For this review, take the finished solid that the model builds, in its own axes (mm). Face numbers are marked on the shaded views. A direction names the side the tool comes from. Round coordinates to 2 decimals unless told otherwise and drop trailing zeros. Loops run counter-clockwise (first coordinate to the right, second up) from the corner with the lowest first, then second, coordinate; pieces in that order, holes last.
1) Insertion check: pin 1 (1 mm diameter, centred on x = 202, y = 166.5, fed in from -Z). The pin has a flat end and moves straight along its axis. Give the tip position at first contact, or say it passes through.
2) Take a section at D-D (y = 178.25). State the section outline as (x, z) points.
3) Take a section at C-C (x = 196). State the section outline as (y, z) points.
4) Wall thickness on L1, parallel to Y at x = 202.5, z = 2.4; L2, parallel to Y at x = 195.5, z = 2.75; L3, parallel to X at y = 174.25, z = 1.45: over which ranges is each line inside the solid? List them lowest first.
5) Take a section at A-A (x = 203.5). State the section outline as (y, z) points.
6) Mouldability with a two-part tool opening along Y and no side actions: class the marked faces 3, 4, 5 and 6 as pulls with the +Y half, pulls with the -Y half, needs draft (parallel to the pull), parting line crosses it, or undercut.
7) Take a section at B-B (z = 1.1). State the section outline as (x, y) points.
8) Tool access review of the marked faces 1 and 2: name each direction out of +Z, -Z, +X, -X, +Y, -Y from which nothing blocks a thin tool from reaching the whole face with its end or side.
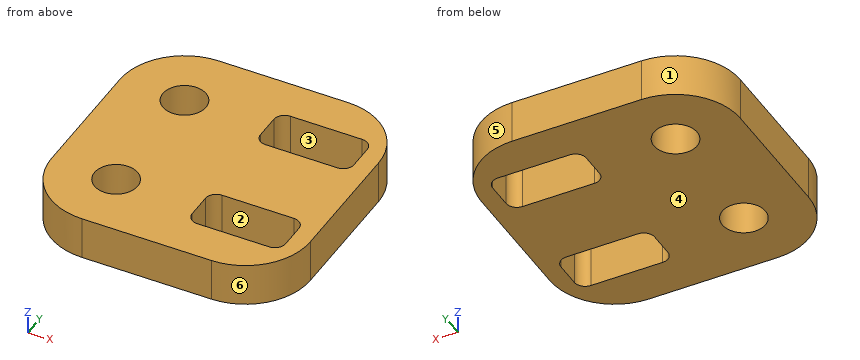
```python
from build123d import *

# Parameters (mm, degrees)
MODEL_R                 = 1.5
SALIENTE_EXTRUIR1_DEPTH = 3


with BuildPart() as part:
    # Model → Saliente-Extruir1 (new body)
    with BuildSketch(Plane.XY):
        with BuildLine():
            Line((195.335922194, 161.333196305), (204.335922194, 161.333196305))
            ThreePointArc((204.335922194, 161.333196305), (207.517902709, 162.651215789), (208.835922194, 165.833196305))
            Line((208.835922194, 165.833196305), (208.835922194, 174.833196305))
            ThreePointArc((208.835922194, 174.833196305), (207.517902709, 178.01517682), (204.335922194, 179.333196305))
            Line((204.335922194, 179.333196305), (195.335922194, 179.333196305))
            ThreePointArc((195.335922194, 179.333196305), (192.153941678, 178.01517682), (190.835922194, 174.833196305))
            Line((190.835922194, 174.833196305), (190.835922194, 165.833196305))
            ThreePointArc((190.835922194, 165.833196305), (192.153941678, 162.651215789), (195.335922194, 161.333196305))
        make_face()
        with Locations((195.335922194, 174.833196305)):
            Circle(MODEL_R, mode=Mode.SUBTRACT)
        with Locations((195.335922194, 165.833196305)):
            Circle(MODEL_R, mode=Mode.SUBTRACT)
        with BuildLine():
            Line((206.835922194, 173.208196305), (201.835922194, 173.208196305))
            ThreePointArc((201.835922194, 173.208196305), (201.305592108, 173.427866219), (201.085922194, 173.958196305))
            Line((201.085922194, 173.958196305), (201.085922194, 175.708196305))
            ThreePointArc((201.085922194, 175.708196305), (201.305592108, 176.23852639), (201.835922194, 176.458196305))
            Line((201.835922194, 176.458196305), (206.835922194, 176.458196305))
            ThreePointArc((206.835922194, 176.458196305), (207.36625228, 176.23852639), (207.585922194, 175.708196305))
            Line((207.585922194, 175.708196305), (207.585922194, 173.958196305))
            ThreePointArc((207.585922194, 173.958196305), (207.36625228, 173.427866219), (206.835922194, 173.208196305))
        make_face(mode=Mode.SUBTRACT)
        with BuildLine():
            Line((206.835922194, 164.208196305), (201.835922194, 164.208196305))
            ThreePointArc((201.835922194, 164.208196305), (201.305592108, 164.427866219), (201.085922194, 164.958196305))
            Line((201.085922194, 164.958196305), (201.085922194, 166.708196305))
            ThreePointArc((201.085922194, 166.708196305), (201.305592108, 167.23852639), (201.835922194, 167.458196305))
            Line((201.835922194, 167.458196305), (206.835922194, 167.458196305))
            ThreePointArc((206.835922194, 167.458196305), (207.36625228, 167.23852639), (207.585922194, 166.708196305))
            Line((207.585922194, 166.708196305), (207.585922194, 164.958196305))
            ThreePointArc((207.585922194, 164.958196305), (207.36625228, 164.427866219), (206.835922194, 164.208196305))
        make_face(mode=Mode.SUBTRACT)
    extrude(amount=SALIENTE_EXTRUIR1_DEPTH)


solid = part.part
```
Response:
1. pin 1: passes through
2. outline: (192.41, 0) - (207.26, 0) - (207.26, 3) - (192.41, 3) - close
3. outline: (161.33, 0) - (164.49, 0) - (164.49, 3) - (161.33, 3) - close; (167.18, 0) - (173.49, 0) - (173.49, 3) - (167.18, 3) - close; (176.18, 0) - (179.33, 0) - (179.33, 3) - (176.18, 3) - close
4. L1: y = 161.33 to 164.21, 167.46 to 173.21, 176.46 to 179.33
4. L2: y = 161.33 to 164.34, 167.32 to 173.34, 176.32 to 179.33
4. L3: x = 190.84 to 193.95, 196.72 to 201.09, 207.59 to 208.84
5. outline: (161.33, 0) - (164.21, 0) - (164.21, 3) - (161.33, 3) - close; (167.46, 0) - (173.21, 0) - (173.21, 3) - (167.46, 3) - close; (176.46, 0) - (179.33, 0) - (179.33, 3) - (176.46, 3) - close
6. face 3: undercut
6. face 4: needs draft
6. face 5: pulls with the +Y half
6. face 6: pulls with the -Y half
7. outline: (190.84, 165.83) arc R4.5 ccw to (195.34, 161.33) - (204.34, 161.33) arc R4.5 ccw to (208.84, 165.83) - (208.84, 174.83) arc R4.5 ccw to (204.34, 179.33) - (195.34, 179.33) arc R4.5 ccw to (190.84, 174.83) - close; hole circle Ø3 at (195.34, 165.83); hole circle Ø3 at (195.34, 174.83); hole (201.09, 164.96) arc R0.75 ccw to (201.84, 164.21) - (206.84, 164.21) arc R0.75 ccw to (207.59, 164.96) - (207.59, 166.71) arc R0.75 ccw to (206.84, 167.46) - (201.84, 167.46) arc R0.75 ccw to (201.09, 166.71) - close; hole (201.09, 173.96) arc R0.75 ccw to (201.84, 173.21) - (206.84, 173.21) arc R0.75 ccw to (207.59, 173.96) - (207.59, 175.71) arc R0.75 ccw to (206.84, 176.46) - (201.84, 176.46) arc R0.75 ccw to (201.09, 175.71) - close
8. face 1: +Z, -Z, -X, +Y
8. face 2: +Z, -Z
